from build123d import *

# Parameters (mm, degrees)
ESQUISSE1_W             = 10
ESQUISSE1_H             = 3
ESQUISSE1_W_2           = 140
ESQUISSE1_H_2           = 75
BOSS_EXTRU_1_DEPTH      = 3
ESQUISSE2_W             = 4
ESQUISSE2_H             = 60
ENL_V_MAT_EXTRU_1_DEPTH = 3


with BuildPart() as part:
    # Esquisse1 → Boss.-Extru.1 (new body)
    with BuildSketch(Plane.XY):
        with Locations((-107.5, -1.5)):
            Rectangle(ESQUISSE1_W, ESQUISSE1_H)
        with Locations((-82.5, -1.5)):
            Rectangle(ESQUISSE1_W, ESQUISSE1_H)
        with Locations((-57.5, -1.5)):
            Rectangle(ESQUISSE1_W, ESQUISSE1_H)
        with Locations((-32.5, -1.5)):
            Rectangle(ESQUISSE1_W, ESQUISSE1_H)
        with Locations((-7.5, -1.5)):
            Rectangle(ESQUISSE1_W, ESQUISSE1_H)
        with Locations((-70, 37.5)):
            Rectangle(ESQUISSE1_W_2, ESQUISSE1_H_2)
        with Locations((-132.5, -1.5)):
            Rectangle(ESQUISSE1_W, ESQUISSE1_H)
    extrude(amount=BOSS_EXTRU_1_DEPTH)

    # Esquisse2 → Enl_v. mat.-Extru.1 (cut)
    with BuildSketch(Plane.XY.offset(3)):
        with Locations((-133, 38)):
            Rectangle(ESQUISSE2_W, ESQUISSE2_H)
        with Locations((-123, 38)):
            Rectangle(ESQUISSE2_W, ESQUISSE2_H)
        with Locations((-113, 38)):
            Rectangle(ESQUISSE2_W, ESQUISSE2_H)
        with Locations((-103, 38)):
            Rectangle(ESQUISSE2_W, ESQUISSE2_H)
        with Locations((-93, 38)):
            Rectangle(ESQUISSE2_W, ESQUISSE2_H)
        with Locations((-83, 38)):
            Rectangle(ESQUISSE2_W, ESQUISSE2_H)
        with Locations((-73, 38)):
            Rectangle(ESQUISSE2_W, ESQUISSE2_H)
        with Locations((-63, 38)):
            Rectangle(ESQUISSE2_W, ESQUISSE2_H)
        with Locations((-53, 38)):
            Rectangle(ESQUISSE2_W, ESQUISSE2_H)
        with Locations((-43, 38)):
            Rectangle(ESQUISSE2_W, ESQUISSE2_H)
        with Locations((-33, 38)):
            Rectangle(ESQUISSE2_W, ESQUISSE2_H)
        with Locations((-23, 38)):
            Rectangle(ESQUISSE2_W, ESQUISSE2_H)
        with Locations((-13, 38)):
            Rectangle(ESQUISSE2_W, ESQUISSE2_H)
    extrude(amount=-ENL_V_MAT_EXTRU_1_DEPTH, mode=Mode.SUBTRACT)


solid = part.part
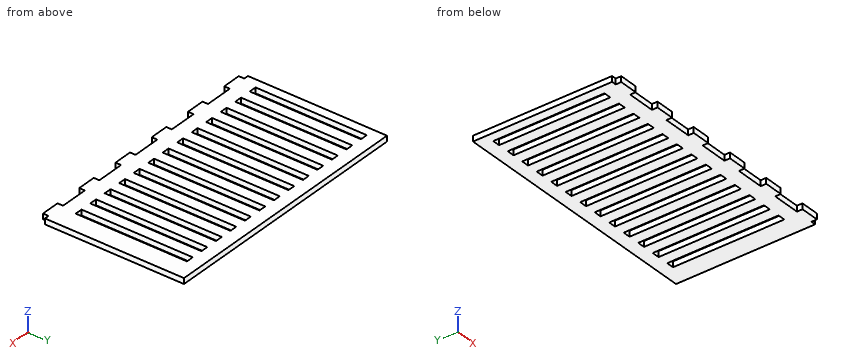
Work out the finished part from the listing and answer in its coordinate system (mm). Coordinates: 2 decimals unless noted, no trailing zeros. Answer as CSV lines item,"result". Start each with the question number.
Item 1: Flat-ended cylindrical pins translate along their axes: P1, Ø1, axis at x = -15.5, z = 2, coming from the -Y side; P2, Ø0.9, axis at y = -1, z = 1, coming from the -X side; P3, Ø0.9, axis at y = 43, z = 2, coming from the +X side. Find the tip coordinate at first contact, or state that the pin passes through.
Item 2: Consider L1, parallel to Y at x = -113, z = 0.55; L2, parallel to Y at x = -62, z = 2.7; L3, parallel to Y at x = -47.5, z = 1.75. Determine where each line is inside the solid, lowest interval first.
Item 3: Section A-A on y = 27 is taken. Give the number of separate pieces and of enclosed holes in the cut face, and give its area (3 significant figures).
Checks:
1,P1,"stops at y = 0"
1,P2,"stops at x = -137.5"
1,P3,"stops at x = 0"
2,L1,"y = 0 to 8, 68 to 75"
2,L2,"y = -3 to 8, 68 to 75"
2,L3,"y = 0 to 75"
3,separate pieces,"14"
3,enclosed holes,"0"
3,area,"264 mm²"
